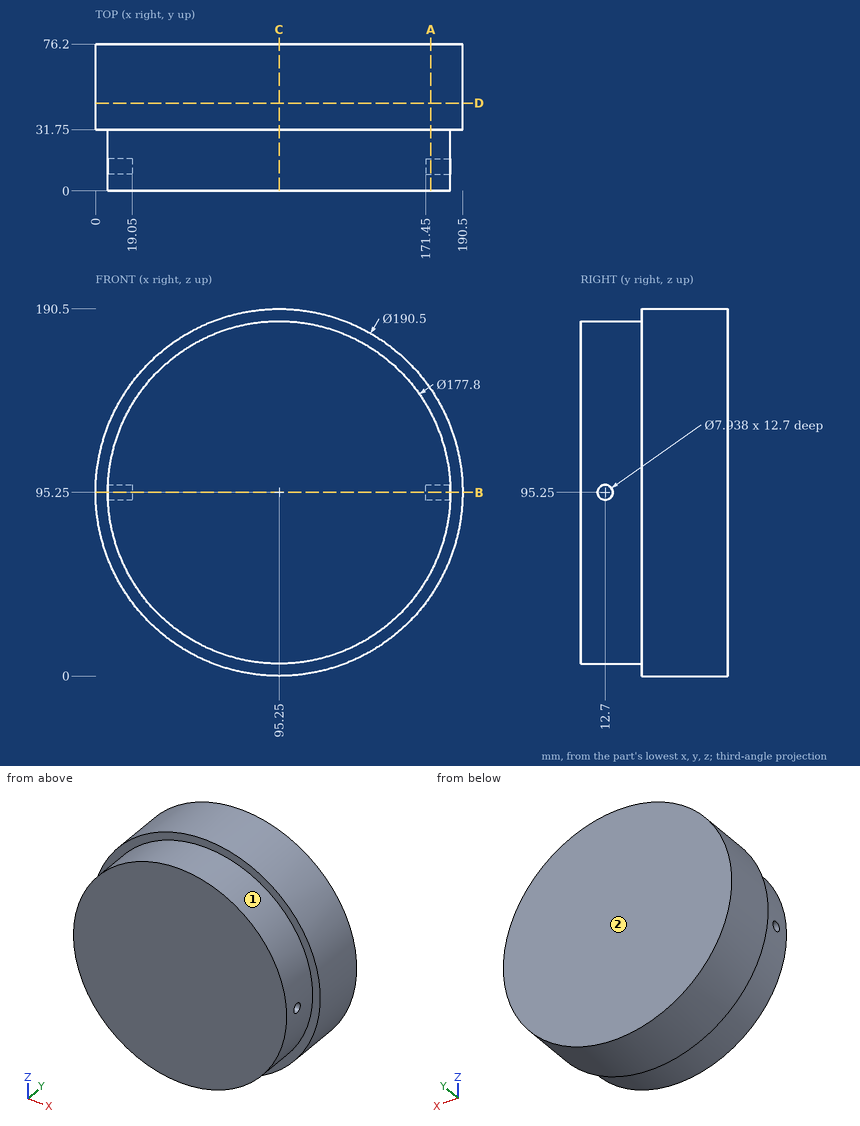
Geometry check sheet. Reference: drawing and pictorial views, mm from the part's lowest x, y, z. A direction names the side the tool comes from. Give positions to 0.01 mm unless a question says otherwise; leave off trailing zeros. Loops run counter-clockwise (first coordinate to the right, second up) from the corner with the lowest first, then second, coordinate; pieces in that order, holes last. Notation, with made-up numbers: M 21.25,68.5 L 52.25,68.5 A20 cw 52.25,101.5 Z; hole C 81.5,-30 d8. An arc over 180 degrees is marked long. Use a Markdown table: item, result. Add a question column.
Q1. Go/stop test with flat-tipped pins: pin 1 (2.5 mm diameter, centred on y = 11.5, z = 95, fed in from +X); pin 2 (5 mm diameter, centred on y = 50, z = 38.5, fed in from -X); pin 3 (1 mm diameter, centred on x = 149.5, y = 41, fed in from +Z) (1 decimal). Record where each tip stops, or that it passes through.
Q2. Sectioned sample at D-D, the plane y = 45.5. Record the cut outline in (x, z).
Q3. Sectioned sample at B-B, the plane z = 95.25. Record the cut outline in (x, y).
Q4. Sectioned sample at A-A, the plane x = 174. Record the cut outline in (y, z), then the cut area to 3 significant figures.
Q5. Sectioned sample at C-C, the plane x = 95.25. Record the cut outline in (y, z), then the cut area to 3 significant figures.
Q6. Scan lines: line 1 along Y through (x, z) = (9, 95); line 2 along X through (y, z) = (5.5, 97.5); line 3 along Z through (x, y) = (16, 12) (1 decimal). Record each from-to range of solid material in increasing order. Write a range as [from, to].
Q7. Tool access check on the marked faces 1 and 2. Record the directions out of +Z, -Z, +X, -X, +Y, -Y that give a thin tool (end or side, any length) a straight path to the whole face; none if there is none.
Verdict:
| question | item | result |
|---|---|---|
| 1 | pin 1 | x = 171.45 |
| 1 | pin 2 | x = 16.96 |
| 1 | pin 3 | z = 173.9 |
| 2 | outline | C 95.25,95.25 d190.5 |
| 3 | outline | M 0,31.75 L 6.35,31.75 L 6.35,16.67 L 19.05,16.67 L 19.05,8.73 L 6.35,8.73 L 6.35,0 L 184.15,0 L 184.15,8.73 L 171.45,8.73 L 171.45,16.67 L 184.15,16.67 L 184.15,31.75 L 190.5,31.75 L 190.5,76.2 L 0,76.2 Z |
| 4 | outline | M 0,54 L 31.75,54 L 31.75,41.67 L 76.2,41.67 L 76.2,148.83 L 31.75,148.83 L 31.75,136.5 L 0,136.5 Z; hole C 12.7,95.25 d7.94 |
| 4 | area | 7,330 mm^2 |
| 5 | outline | M 0,6.35 L 31.75,6.35 L 31.75,0 L 76.2,0 L 76.2,190.5 L 31.75,190.5 L 31.75,184.15 L 0,184.15 Z |
| 5 | area | 14,100 mm^2 |
| 6 | line 1 | [0, 8.74], [16.66, 76.2] |
| 6 | line 2 | [6.38, 184.12] |
| 6 | line 3 | [55, 91.3], [99.2, 135.5] |
| 7 | face 1 | -Y |
| 7 | face 2 | +Z, -Z, +X, -X, +Y |
